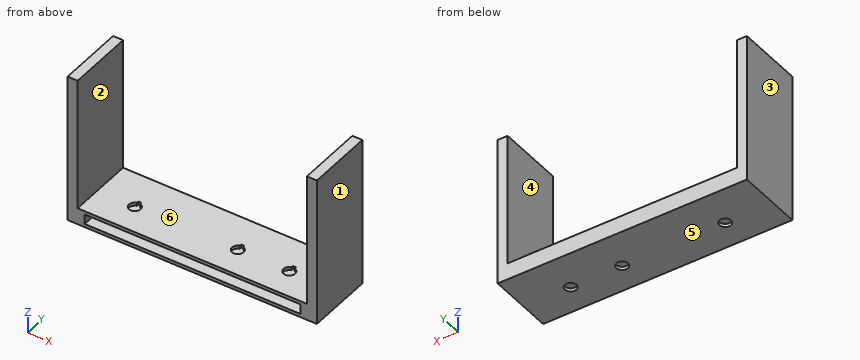
```python
from build123d import *

# Parameters (mm, degrees)
SKETCH1_W           = 150
SKETCH1_H           = 40
BOSS_EXTRUDE1_DEPTH = 10
SKETCH2_W           = 130
SKETCH2_H           = 6
CUT_EXTRUDE1_DEPTH  = 34
CUT_EXTRUDE3_DEPTH  = 10
BOSS_EXTRUDE2_DEPTH = 2
SKETCH5_W           = 6
SKETCH5_H           = 40
BOSS_EXTRUDE3_DEPTH = 80


with BuildPart() as part:
    # Sketch1 → Boss-Extrude1 (new body)
    with BuildSketch(Plane.XY):
        Rectangle(SKETCH1_W, SKETCH1_H)
    extrude(amount=BOSS_EXTRUDE1_DEPTH)

    # Sketch2 → Cut-Extrude1 (cut)
    with BuildSketch(Plane.XZ.offset(20)):
        with Locations((0.265824487, 5)):
            Rectangle(SKETCH2_W, SKETCH2_H)
    extrude(amount=-CUT_EXTRUDE1_DEPTH, mode=Mode.SUBTRACT)

    # Sketch3 → Cut-Extrude3 (cut)
    with BuildSketch(Plane.XY.offset(10)):
        with BuildLine():
            Line((16.765824487, 1.504101966), (16.765824487, 0.354101966))
            ThreePointArc((16.765824487, 0.354101966), (15.765824487, -6.5), (14.765824487, 0.354101966))
            Line((14.765824487, 0.354101966), (14.765824487, 1.504101966))
            Line((14.765824487, 1.504101966), (16.765824487, 1.504101966))
        make_face()
        with BuildLine():
            Line((-45.234175513, 1.504101966), (-47.234175513, 1.504101966))
            Line((-47.234175513, 1.504101966), (-47.234175513, 0.354101966))
            ThreePointArc((-47.234175513, 0.354101966), (-46.234175513, -6.5), (-45.234175513, 0.354101966))
            Line((-45.234175513, 0.354101966), (-45.234175513, 1.504101966))
        make_face()
        with BuildLine():
            Line((47.765824487, 1.504101966), (47.765824487, 0.354101966))
            ThreePointArc((47.765824487, 0.354101966), (46.765824487, -6.5), (45.765824487, 0.354101966))
            Line((45.765824487, 0.354101966), (45.765824487, 1.504101966))
            Line((45.765824487, 1.504101966), (47.765824487, 1.504101966))
        make_face()
    extrude(amount=-CUT_EXTRUDE3_DEPTH, mode=Mode.SUBTRACT)

    # Sketch4 → Boss-Extrude2 (add)
    with BuildSketch(Plane(origin=(0, 0, 0), x_dir=(-1, 0, 0), z_dir=(0, 0, -1))):
        with BuildLine():
            Line((-47.765824487, 0.354101966), (-47.765824487, 1.504101966))
            Line((-47.765824487, 1.504101966), (-45.765824487, 1.504101966))
            Line((-45.765824487, 1.504101966), (-45.765824487, 0.354101966))
            ThreePointArc((-45.765824487, 0.354101966), (-46.765824487, 0.5), (-47.765824487, 0.354101966))
        make_face()
        with BuildLine():
            Line((-14.765824487, 1.504101966), (-14.765824487, 0.354101966))
            ThreePointArc((-14.765824487, 0.354101966), (-15.765824487, 0.5), (-16.765824487, 0.354101966))
            Line((-16.765824487, 0.354101966), (-16.765824487, 1.504101966))
            Line((-16.765824487, 1.504101966), (-14.765824487, 1.504101966))
        make_face()
        with BuildLine():
            Line((47.234175513, 1.504101966), (47.234175513, 0.354101966))
            ThreePointArc((47.234175513, 0.354101966), (46.234175513, 0.5), (45.234175513, 0.354101966))
            Line((45.234175513, 0.354101966), (45.234175513, 1.504101966))
            Line((45.234175513, 1.504101966), (47.234175513, 1.504101966))
        make_face()
    extrude(amount=-BOSS_EXTRUDE2_DEPTH)

    # Sketch5 → Boss-Extrude3 (add)
    with BuildSketch(Plane.XY.offset(10)):
        with Locations((-72, 0)):
            Rectangle(SKETCH5_W, SKETCH5_H)
        with Locations((72, 0)):
            Rectangle(SKETCH5_W, SKETCH5_H)
    extrude(amount=BOSS_EXTRUDE3_DEPTH)


solid = part.part
```
The listing builds one solid part. Answer for the finished solid, in the listing's coordinates (mm). Face numbers are marked on the shaded views. A direction names the side the tool comes from. Give positions to 0.01 mm unless a question says otherwise; leave off trailing zeros. Order: outer loops, then holes, each group sorted by start corner. A loop starts at its lowest first (then second) coordinate and runs counter-clockwise, first axis right, second up. Notation, with made-up numbers: M -8,22.5 L 22,22.5 A23 cw 22,47.5 Z; hole C 29.25,-21 d7. An arc over 180 degrees is marked long. Put each result on its own line as item: value. Start each with the question number.
Item 1: Flat-ended cylindrical pins translate along their axes: P1, Ø1.8, axis at x = -24.5, z = 4.5, coming from the -Y side; P2, Ø12, axis at x = 5.5, y = 2, coming from the +Z side. Find the tip coordinate at first contact, or state that the pin passes through.
Item 2: For a pull along X with two mould halves and no side action, classify the marked faces 3, 4, 5 and 6 as +X half, -X half, draft (parallel to the pull), parting line (faces both ways), or undercut.
Item 3: The part is cut by section B-B, the plane y = 7.5. Determine the outline of the cut face in (x, z).
Item 4: The part is cut by section A-A, the plane z = 33. Determine the outline of the cut face in (x, y), and give its area (3 significant figures).
Item 5: The part is cut by section D-D, the plane y = -3. State how many separate pieces and enclosed holes the cut face has, and give its area (3 significant figures).
Item 6: The part is cut by section C-C, the plane x = 22. Determine the outline of the cut face in (y, z), and give its area (3 significant figures).
Item 7: Which of the six approach directions +Z, -Z, +X, -X, +Y, -Y give full straight-line access (tool end or side, diameter ignored) to the marked faces 1 and 2?
Item 8: Find the intervals of material crossed by line 1 along X through (y, z) = (-3, 8.85); line 2 along Z through (x, y) = (-40, -4.5); line 3 along X through (y, z) = (-17, 38.5), in increasing order.
Answer key:
1. P1: stops at y = 14
1. P2: stops at z = 10
2. face 3: -X half
2. face 4: undercut
2. face 5: draft
2. face 6: undercut
3. outline: M -75,0 L 75,0 L 75,90 L 69,90 L 69,10 L -69,10 L -69,90 L -75,90 Z; hole M -64.73,2 L 65.27,2 L 65.27,8 L -64.73,8 Z
4. outline: M -75,-20 L -69,-20 L -69,20 L -75,20 Z; M 69,-20 L 75,-20 L 75,20 L 69,20 Z
4. area: 480 mm²
5. separate pieces: 6
5. enclosed holes: 0
5. area: 1,600 mm²
6. outline: M -20,0 L 20,0 L 20,10 L -20,10 L -20,8 L 14,8 L 14,2 L -20,2 Z
6. area: 196 mm²
7. face 1: +Z, -Z, +X, +Y, -Y
7. face 2: +Z, +Y, -Y
8. line 1: x = -75 to -49.73, -42.73 to 12.27, 19.27 to 43.27, 50.27 to 75
8. line 2: z = 0 to 2, 8 to 10
8. line 3: x = -75 to -69, 69 to 75
